from build123d import *

# Parameters (mm, degrees)
SKETCH_R           = 7.5
PAD_DEPTH          = 5
SKETCH001_R        = 1
POCKET_DEPTH       = 3
PAD001_DEPTH       = 5
POLARPATTERN_COUNT = 20


with BuildPart() as part:
    # Sketch → Pad (new body)
    with BuildSketch(Plane.YZ):
        Circle(SKETCH_R)
    extrude(amount=PAD_DEPTH)

    # Sketch001 (on Face3 of Pad) → Pocket (cut)
    with BuildSketch(Plane.YZ.offset(5)):
        Circle(SKETCH001_R)
    extrude(amount=-POCKET_DEPTH, mode=Mode.SUBTRACT)

    # Sketch002 (on DatumPlane) → Pad001 (join, symmetric)
    with BuildSketch(Plane.ZX.offset(7.5)):
        Polygon((0.8, 0.3), (-0.3, 5), (-0.8, 5), (0.3, 0.3), align=None)
    pad001 = extrude(amount=PAD001_DEPTH, both=True)

    # PolarPattern: Pad001 ×20 about axis
    polarpattern_axis = Axis((0, 0, 0), (1, 0, 0))
    for i in range(1, POLARPATTERN_COUNT):
        add(pad001.rotate(polarpattern_axis, i * 360 / POLARPATTERN_COUNT))


solid = part.part
For this review, take the finished solid that the model builds, in its own axes (mm). A direction names the side the tool comes from. Give positions to 0.01 mm unless a question says otherwise; leave off trailing zeros. Order: outer loops, then holes, each group sorted by start corner. A loop starts at its lowest first (then second) coordinate and runs counter-clockwise, first axis right, second up. Notation, with made-up numbers: M 17,-7.5 L 47,-7.5 A15 ccw 47,11.5 Z; hole C 14,-14 d5. An arc over 180 degrees is marked long. Answer in a Markdown table with one row per item. Add a question column.
(1) Wall thickness on probe 1 along Z at (x, y) = (0.75, -8); probe 2 along Y at (x, z) = (1.8, 5); probe 3 along Z at (x, y) = (1.8, -10): over which ranges is each line inside the solid? List them lowest first. Write a range as [from, to].
(2) Consider section B-B on y = 0. State the section outline as (x, z) points, and give its area (3 significant figures).
(3) For faces 1 (the face through (0.3, 8.4, -5.4)), 2 (the face through (2.617, 6.095, -7.95)), 3 (the face through (2.617, -8.253, 5.678)), 4 (the face through (2.683, -6.095, -7.95)), list the 3-axis set-ups (+Z, -Z, +X, -X, +Y, -Y) from which the entire face can be reached by the end or side of a thin tool; tool diameter is ignored.
(4) Mouldability with a two-part tool opening along Y and no side actions: class faces 5 (the face through (2.683, 10.014, -0.258)), 6 (the face through (2.683, 6.095, 7.95)), 7 (the face through (4, 0, -1)), 8 (the face through (2.661, -11.905, 3.81)) as +Y half, -Y half, draft (parallel to the pull), parting line (faces both ways), or undercut.
(5) For pin 1 (3 mm diameter, centred on y = -4, z = 8.5, fed in from +X); pin 2 (1.5 mm diameter, centred on x = 3, z = -6.5, fed in from -Y); pin 3 (1.5 mm diameter, centred on x = 1, y = 7.5, fed in from -Z); pin 4 (1.6 mm diameter, centred on y = 10.5, z = -2.5, fed in from -X), all flat-tipped, find the tip position at first contact; note any pin that passes through.
(6) Consider section A-A on z = -8.5. State the section outline as (x, y) points, and give its area (3 significant figures).
Evaluation:
| question | item | result |
|---|---|---|
| 1 | probe 1 | z = [-6.67, -6.05], [-3.33, -2.8], [-0.69, -0.19], [1.87, 2.39], [4.95, 5.57] |
| 1 | probe 2 | y = [-7.65, -6.8], [-5.59, 5.59], [6.12, 6.97] |
| 1 | probe 3 | z = [-7.5, -7.2], [-3.72, -3.2], [-0.45, 0.05], [2.78, 3.3], [6.71, 7.33] |
| 2 | outline | M 0,-7.5 L 1.58,-7.5 L 1.58,-12.5 L 3.72,-12.5 L 3.72,-7.5 L 5,-7.5 L 5,-1 L 2,-1 L 2,1 L 5,1 L 5,7.5 L 3.72,7.5 L 3.72,12.5 L 1.58,12.5 L 1.58,7.5 L 0,7.5 Z |
| 2 | area | 90.4 mm^2 |
| 3 | face 1 | -Z, -X, +Y |
| 3 | face 2 | +X |
| 3 | face 3 | +X, -Y |
| 3 | face 4 | -X |
| 4 | face 5 | draft |
| 4 | face 6 | undercut |
| 4 | face 7 | undercut |
| 4 | face 8 | -Y half |
| 5 | pin 1 | stops at x = 5 |
| 5 | pin 2 | stops at y = -10.39 |
| 5 | pin 3 | stops at z = -10.13 |
| 5 | pin 4 | stops at x = 0.3 |
| 6 | outline | M 0.3,-5.8 L 5,-7.16 L 5,-6.55 L 0.3,-5.19 Z; M 0.3,-2.45 L 5,-3.6 L 5,-3.08 L 0.3,-1.92 Z; M 0.3,0.3 L 5,-0.8 L 5,-0.3 L 0.3,0.8 Z; M 0.3,3.08 L 5,1.92 L 5,2.45 L 0.3,3.6 Z; M 0.3,6.55 L 5,5.19 L 5,5.8 L 0.3,7.16 Z |
| 6 | area | 13.1 mm^2 |
